Answer from the drawing. Dimensions are ordinates in mm from the lowest x, y and z of the part. A direction names the side the tool comes from. Give positions to 0.01 mm unless a question says otherwise; leave off trailing zeros. Order: outer loops, then holes, each group sorted by start corner. A loop starts at its lowest first (then second) coordinate and runs counter-clockwise, first axis right, second up. Notation, with made-up numbers: (53, 79.25) - (97, 79.25) arc R20 cw to (97, 114.25) - close; hole circle Ø4 at (60.5, 73). An arc over 180 degrees is marked (long way). Use a Markdown table: item, result. Add a question column.
1) Straight lines are drawn through the part: line 1 (Y direction, x = 7.5, z = 1.5) (1 decimal); line 2 (X direction, y = 7.5, z = 1.1) (1 decimal); line 3 (X direction, y = 30, z = 42). For each, find the intervals that lie inside material, in ascending order.
2) For the marked faces 1, 2, 3, 4 and 5, determine the directions among +Z, -Z, +X, -X, +Y, -Y from which every point of the face is accessible in a straight line to the end or side of a thin tool.
3) Find section D-D, the plane z = 33.5. Determine the outline of the cut face in (x, y).
4) Find section B-B, the plane y = 7.5. Determine the outline of the cut face in (x, z) (1 decimal).
5) Find section A-A, the plane x = 7.5. State how many separate pieces and enclosed holes the cut face has, plus the area to 3 significant figures.
6) Flat-ended cylindrical pins translate along their axes: pin 1 (2 mm diameter, centred on x = 2.5, z = 18.5, fed in from +Y); pin 2 (0.8 mm diameter, centred on x = 2.5, z = 19.5, fed in from -Y); pin 3 (3 mm diameter, centred on y = 25, z = 38.5, fed in from +X). Find the tip coordinate at first contact, or state that the pin passes through.
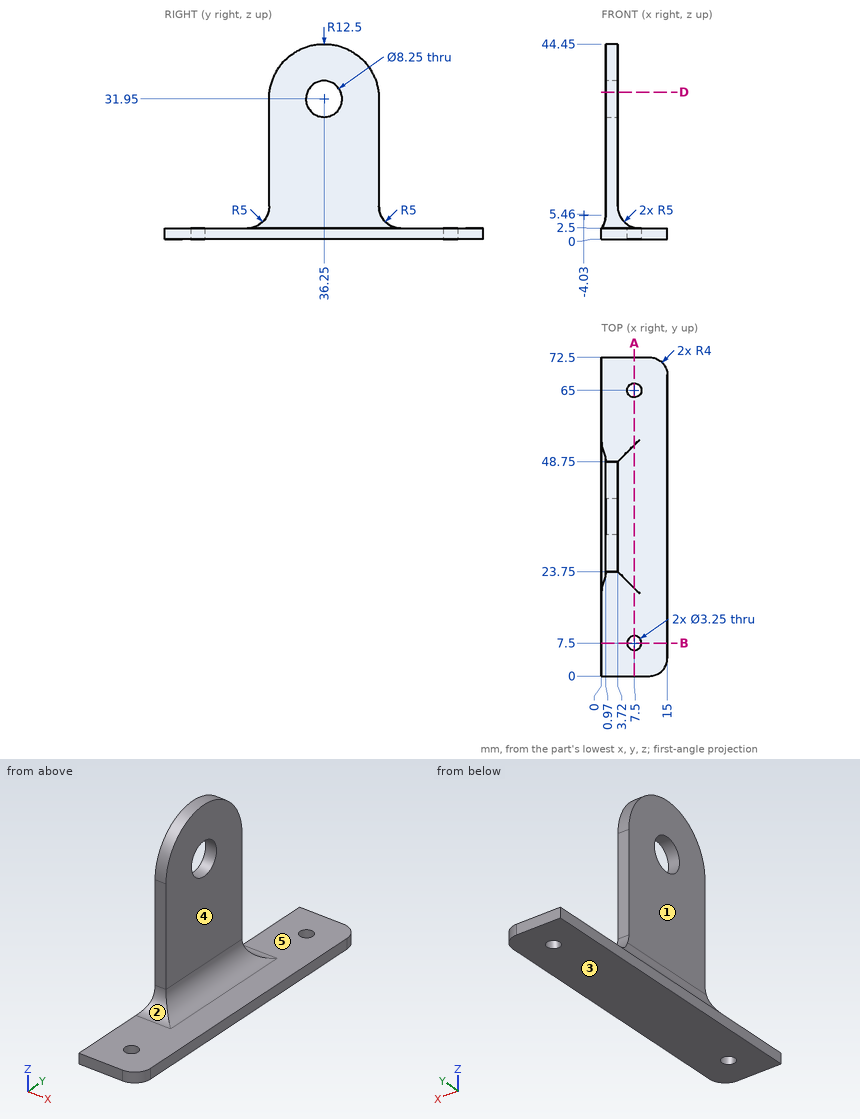
The answers:
| question | item | result |
|---|---|---|
| 1 | line 1 | 0 to 5.9, 9.1 to 63.4, 66.6 to 72.5 |
| 1 | line 2 | 0 to 5.9, 9.1 to 15 |
| 1 | line 3 | 0.97 to 3.72 |
| 2 | face 1 | +Z, -X, +Y, -Y |
| 2 | face 2 | +Z, +X, -X, -Y |
| 2 | face 3 | -Z, +X, -X, +Y, -Y |
| 2 | face 4 | +Z, +X, +Y, -Y |
| 2 | face 5 | +Z, +X |
| 3 | outline | (0.97, 23.85) - (3.72, 23.85) - (3.72, 32.43) - (0.97, 32.43) - close; (0.97, 40.07) - (3.72, 40.07) - (3.72, 48.65) - (0.97, 48.65) - close |
| 4 | outline | (0, 0) - (5.9, 0) - (5.9, 2.5) - (0, 2.5) - close; (9.1, 0) - (15, 0) - (15, 2.5) - (9.1, 2.5) - close |
| 5 | separate pieces | 3 |
| 5 | enclosed holes | 0 |
| 5 | area | 170 mm2 |
| 6 | pin 1 | y = 48.75 |
| 6 | pin 2 | y = 23.75 |
| 6 | pin 3 | x = 3.72 |
